from build123d import *

# Parameters (mm, degrees)
CUT_EXTRUDE1_DEPTH = 2.2
CHAMFER1_SIZE      = 0.5


with BuildPart() as part:
    # Sketch1 → Revolve1 (revolve)
    with BuildSketch(Plane.XY):
        Polygon((0, 0), (0, 5.67), (-1.05, 5.67), (-3.72, 3), (-20, 3), (-20, 0), align=None)
    revolve(axis=Axis((0, 0, 0), (-1, 0, 0)))

    # Sketch2 → Cut-Extrude1 (cut)
    with BuildSketch(Plane(origin=(0, 0, 0), x_dir=(0, 0, -1), z_dir=(1, 0, 0))):
        Polygon((2.309401077, 0), (1.154700538, 2), (-1.154700538, 2), (-2.309401077, 0), (-1.154700538, -2), (1.154700538, -2), align=None)
    extrude(amount=-CUT_EXTRUDE1_DEPTH, mode=Mode.SUBTRACT)

    # Chamfer1
    chamfer1_edges = [part.edges().sort_by_distance(p)[0] for p in [
        (-20, -3, 0),
    ]]
    chamfer(chamfer1_edges, length=CHAMFER1_SIZE)


solid = part.part
The listing builds one solid part. Answer for the finished solid, in the listing's coordinates (mm). A direction names the side the tool comes from. Round coordinates to 2 decimals unless told otherwise and drop trailing zeros. Loops run counter-clockwise (first coordinate to the right, second up) from the corner with the lowest first, then second, coordinate; pieces in that order, holes last. Notation, with made-up numbers: M 24.5,-17.5 L 52.5,-17.5 A12 cw 52.5,3.5 Z; hole C 31.5,16.5 d5. An arc over 180 degrees is marked long. Write each question's results on one line, items separated by ' | '. Start each with the question number.
1) Find section B-B on z = 0. Write down the section's boundary in (x, y), plus the area to 3 significant figures.
2) Each of these flat-tipped pins is pushed along its axis until it touches: pin 1 (1 mm diameter, centred on x = -17, y = 0, fed in from -Z); pin 2 (5 mm diameter, centred on x = -13, z = 0.5, fed in from -Y); pin 3 (1 mm diameter, centred on y = 1.5, z = -3, fed in from -X). Where does it stop, or does it pass through?
3) Find section C-C on x = -10. Write down the section's boundary in (y, z).
4) Determine the mould class of faces 1 (the flat face through (0, -2.4, -0.1)), 2 (the cylindrical face through (-0.53, -0.74, -5.62)), 3 (the flat face through (-1.085, -1.014, -1.724)) for opening direction Z: pulls with the +Z half, pulls with the -Z half, needs draft (parallel to the pull), parting line crosses it, or undercut.
5) Find section A-A on x = -1.5. Write down the section's boundary in (y, z).
6) Straight lines are drawn through the part: probe 1 along Y at (x, z) = (-7.25, 0); probe 2 along Y at (x, z) = (-1.75, 2); probe 3 along Z at (x, y) = (-1.25, 0.75). For each, find the intervals that lie inside material, in ascending order.
7) Which of the six approach directions +Z, -Z, +X, -X, +Y, -Y give full straight-line access (tool end or side, diameter ignored) to faces 4 (the flat face through (-20, 0, 0)), 5 (the flat face through (-1.08, -0.99, 1.74)), 6 (the cylindrical face through (-12, -3, 0))?
Final values:
1) outline: M -20,-2.5 L -19.5,-3 L -3.72,-3 L -1.05,-5.67 L 0,-5.67 L 0,-2 L -2.2,-2 L -2.2,2 L 0,2 L 0,5.67 L -1.05,5.67 L -3.72,3 L -19.5,3 L -20,2.5 Z | area: 124 mm²
2) pin 1: z = -3 | pin 2: y = -3 | pin 3: x = -19.65
3) outline: C 0,0 d6
4) face 1: needs draft | face 2: parting line crosses it | face 3: undercut
5) outline: C 0,0 d10.44; hole M -2,-1.15 L 0,-2.31 L 2,-1.15 L 2,1.15 L 0,2.31 L -2,1.15 Z
6) probe 1: -3 to 3 | probe 2: -4.55 to -0.54, 0.54 to 4.55 | probe 3: -5.42 to -1.88, 1.88 to 5.42
7) face 4: +Z, -Z, -X, +Y, -Y | face 5: +X | face 6: -X
